The listing builds one solid part. Answer for the finished solid, in the listing's coordinates (mm). Face numbers are marked on the shaded views. A direction names the side the tool comes from. Give positions to 0.01 mm unless a question says otherwise; leave off trailing zeros. Write each loop counter-clockwise with the first axis right and the second up, starting at its lowest first coordinate (ties: lowest second). Pieces come first, ordered by that corner, then holes. Notation, with made-up numbers: (43, -23) - (97, -23) arc R12 ccw to (97, -6) - close; hole circle Ø2 at (-14, 8.25). An arc over 180 degrees is marked (long way). Use a Markdown table: item, result. Add a question column.
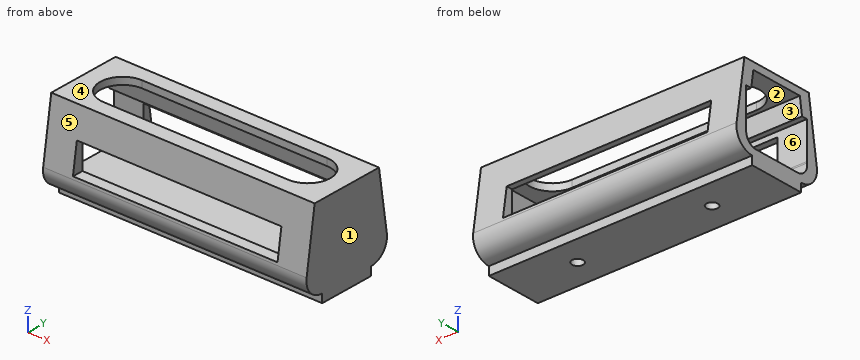
from build123d import *

# Parameters (mm, degrees)
BOSS_EXTRUDE4_DEPTH      = 47
BOSS_EXTRUDE4_DEPTH_BACK = 47
CUT_EXTRUDE1_DEPTH       = 46
CUT_EXTRUDE1_DEPTH_BACK  = 57.471725617
CUT_EXTRUDE2_DEPTH       = 58.688817922
CUT_EXTRUDE2_DEPTH_BACK  = 2.5
CUT_EXTRUDE3_DEPTH       = 57.471725617
CUT_EXTRUDE3_DEPTH_BACK  = 57.471725617
SKETCH22_W               = 73
SKETCH22_H               = 10.4
CUT_EXTRUDE6_DEPTH       = 93
BOSS_EXTRUDE5_START      = -47
SKETCH27_W               = 3
SKETCH27_H               = 20.116454501
BOSS_EXTRUDE5_DEPTH      = 94
SKETCH28_R               = 2
CUT_EXTRUDE7_DEPTH       = 4


with BuildPart() as part:
    # Sketch20 → Boss-Extrude4 (new, two sides: drawn at the far end of the back side and taken through both)
    with BuildSketch(Plane(origin=(0, 0, 0), x_dir=(0, 0, -1), z_dir=(1, 0, 0)).offset(-BOSS_EXTRUDE4_DEPTH_BACK)):
        with BuildLine():
            Line((-26.538783814, 13.222085074), (-26.538783814, -13.211554854))
            Line((-26.538783814, -13.211554854), (-4.989273697, -16.529961404))
            ThreePointArc((-4.989273697, -16.529961404), (0.232004311, -15.039256896), (2.5, -10.105684203))
            Line((2.5, -10.105684203), (2.5, 10.010770298))
            ThreePointArc((2.5, 10.010770298), (0.243783068, 14.93421475), (-4.958555469, 16.439702667))
            Line((-4.958555469, 16.439702667), (-26.538783814, 13.222085074))
        make_face()
    extrude(amount=BOSS_EXTRUDE4_DEPTH + BOSS_EXTRUDE4_DEPTH_BACK)

    # Sketch19 → Cut-Extrude1 (cut, two sides: drawn at the far end of the back side and taken through both)
    with BuildSketch(Plane(origin=(0, 0, 0), x_dir=(0, 0, -1), z_dir=(1, 0, 0)).offset(-CUT_EXTRUDE1_DEPTH_BACK)):
        with BuildLine():
            Line((-24.038783814, 9.55061834), (-4.588783814, 12.45061834))
            ThreePointArc((-4.588783814, 12.45061834), (-1.422994415, 11.554530734), (0, 8.58800374))
            Line((0, 8.58800374), (0, -8.58800374))
            ThreePointArc((0, -8.58800374), (-1.395689655, -11.624048474), (-4.608783814, -12.541405094))
            Line((-4.608783814, -12.541405094), (-24.038783814, -9.54938166))
            Line((-24.038783814, -9.54938166), (-24.038783814, 9.55061834))
        make_face()
    extrude(amount=CUT_EXTRUDE1_DEPTH + CUT_EXTRUDE1_DEPTH_BACK, mode=Mode.SUBTRACT)

    # Sketch21 → Cut-Extrude2 (cut, two sides: drawn at the far end of the back side and taken through both)
    with BuildSketch(Plane.XY.offset(26.538783814).offset(-CUT_EXTRUDE2_DEPTH_BACK)):
        with BuildLine():
            Line((-32.999961179, 8.05061834), (33.000038821, 8.05061834))
            ThreePointArc((33.000038821, 8.05061834), (41.000038821, 0.05061834), (33.000038821, -7.94938166))
            Line((33.000038821, -7.94938166), (-32.999961179, -7.94938166))
            ThreePointArc((-32.999961179, -7.94938166), (-40.999961179, 0.05061834), (-32.999961179, 8.05061834))
        make_face()
    extrude(amount=CUT_EXTRUDE2_DEPTH + CUT_EXTRUDE2_DEPTH_BACK, mode=Mode.SUBTRACT)

    # Sketch22 → Cut-Extrude3 (cut, two sides: drawn at the far end of the back side and taken through both)
    with BuildSketch(Plane(origin=(0, 0, 0), x_dir=(1, 0, 0), z_dir=(0, 1, 0)).offset(-CUT_EXTRUDE3_DEPTH_BACK)):
        with Locations((0, -11.108783814)):
            Rectangle(SKETCH22_W, SKETCH22_H)
    extrude(amount=CUT_EXTRUDE3_DEPTH + CUT_EXTRUDE3_DEPTH_BACK, mode=Mode.SUBTRACT)

    # Sketch26 → Cut-Extrude6 (cut)
    with BuildSketch(Plane.ZY.offset(-46)):
        Polygon((18.098783814, -10.464081567), (18.098783814, -12.474081567), (3.628783814, -12.474081567), (3.66965086, 12.536273867), (18.098783814, 12.536273867), (18.098783814, 10.436273867), align=None)
    extrude(amount=CUT_EXTRUDE6_DEPTH, mode=Mode.SUBTRACT)

    # Sketch27 → Boss-Extrude5 (add)
    with BuildSketch(Plane(origin=(0, 0, 0), x_dir=(0, 0, -1), z_dir=(1, 0, 0)).offset(BOSS_EXTRUDE5_START)):
        with Locations((4, -0.047456953)):
            Rectangle(SKETCH27_W, SKETCH27_H)
    extrude(amount=BOSS_EXTRUDE5_DEPTH)

    # Sketch28 → Cut-Extrude7 (cut)
    with BuildSketch(Plane(origin=(0, 0, -5.5), x_dir=(-1, 0, 0), z_dir=(0, 0, -1))):
        with Locations(Location((-24, 0, 0), (0, 0, 90))):
            Circle(SKETCH28_R)
        with Locations(Location((24, 0, 0), (0, 0, 90))):
            Circle(SKETCH28_R)
    extrude(amount=-CUT_EXTRUDE7_DEPTH, mode=Mode.SUBTRACT)


solid = part.part
1. The part is cut by section C-C (y = 0). Give the vertices of the cut face in (x, z).
2. The part is cut by section A-A (x = -14). Count the separate pieces of the cut face and the enclosed holes in it, and give its area (3 significant figures).
3. Consider L1, parallel to X at y = 0, z = -2; L2, parallel to Z at x = 42.5, y = 0; L3, parallel to X at y = 5.5, z = 1. Determine where each line is inside the solid, lowest interval first. Write a range as [from, to].
4. Which of the six approach directions +Z, -Z, +X, -X, +Y, -Y give full straight-line access (tool end or side, diameter ignored) to the marked faces 5 and 6?
5. The part is cut by section D-D (x = -38.5). Give the vertices of the cut face in (y, z).
6. Given P1, Ø2.5, axis at x = -1, z = -4.5, coming from the +Y side; P2, Ø12, axis at x = -5.5, y = 11.5, coming from the -Z side; P3, Ø3.5, axis at x = 24, y = 0, coming from the -Z side; P4, Ø2.5, axis at x = -2, y = -13.5, coming from the -Z side, each flat-ended and moving along its own axis, determine where each tip first touches the part or whether it passes through.
7. The part is cut by section B-B (z = 10). Give the vertices of the cut face in (x, y), and give its area (3 significant figures).
8. For a pull along Z with two mould halves and no side action, classify the marked faces 1, 2, 3 and 4 as released by +Z, released by -Z, zero draft, split by the parting line, or undercut.
Check values:
| question | item | result |
|---|---|---|
| 1 | outline | (-47, -5.5) - (-26, -5.5) - (-26, -1.5) - (-22, -1.5) - (-22, -5.5) - (22, -5.5) - (22, -1.5) - (26, -1.5) - (26, -5.5) - (47, -5.5) - (47, 26.54) - (41, 26.54) - (41, 24.04) - (46, 24.04) - (46, 0) - (-47, 0) - close; (-47, 24.04) - (-41, 24.04) - (-41, 26.54) - (-47, 26.54) - close |
| 2 | separate pieces | 3 |
| 2 | enclosed holes | 0 |
| 2 | area | 262 mm2 |
| 3 | L1 | x = [-47, -26], [-22, 22], [26, 47] |
| 3 | L2 | z = [-5.5, 0], [24.04, 26.54] |
| 3 | L3 | x = [46, 47] |
| 4 | face 5 | +Z, +X, -X, -Y |
| 4 | face 6 | -X |
| 5 | outline | (-16.53, 4.99) arc R6.5 ccw to (-10.11, -2.5) - (-10.11, -5.5) - (10.01, -5.5) - (10.01, -2.5) arc R6.5 ccw to (16.44, 4.96) - (13.22, 26.54) - (5.86, 26.54) - (5.86, 24.04) - (9.55, 24.04) - (10.44, 18.1) - (12.54, 18.1) - (12.54, 3.67) - (12.48, 3.67) arc R4 cw to (8.59, 0) - (-8.59, 0) arc R4 cw to (-12.54, 4.61) - (-12.47, 5.05) - (-12.47, 18.1) - (-10.46, 18.1) - (-9.55, 24.04) - (-5.76, 24.04) - (-5.76, 26.54) - (-13.21, 26.54) - close |
| 6 | P1 | stops at y = 10.01 |
| 6 | P2 | stops at z = -5.5 |
| 6 | P3 | stops at z = -1.5 |
| 6 | P4 | stops at z = -2.14 |
| 7 | outline | (-47, -15.76) - (-36.5, -15.76) - (-36.5, -12.47) - (-47, -12.47) - close; (-47, 12.54) - (-36.5, 12.54) - (-36.5, 15.69) - (-47, 15.69) - close; (36.5, -15.76) - (47, -15.76) - (47, 15.69) - (36.5, 15.69) - (36.5, 12.54) - (46, 12.54) - (46, -12.47) - (36.5, -12.47) - close |
| 7 | area | 160 mm2 |
| 8 | face 1 | zero draft |
| 8 | face 2 | undercut |
| 8 | face 3 | undercut |
| 8 | face 4 | released by +Z |
